Geometry check sheet. Reference: drawing and pictorial views, mm from the part's lowest x, y, z. A direction names the side the tool comes from. Coordinates: 2 decimals unless noted, no trailing zeros. Loops run counter-clockwise (first coordinate to the right, second up) from the corner with the lowest first, then second, coordinate; pieces in that order, holes last. Notation, with made-up numbers: (-11.5, -3.75) -> (46.5, -3.75) arc R25 cw to (46.5, 18.25) -> close; hole circle Ø9 at (64, 37.5). An arc over 180 degrees is marked (long way). Answer as a JSON object with one key per item and string values. Group by question number.
Q1. Cross-section at B-B on z = 5.5. Record the boundary of the cut face in (x, y).
Q2. Set-up check for the marked faces 1, 2, 3, 4 and 5: record each of +Z, -Z, +X, -X, +Y, -Y from which the full face is reachable in a straight line by a thin tool's end or side.
Q3. Cross-section at C-C on x = 25. Record the boundary of the cut face in (y, z).
Q4. Cross-section at A-A on y = 30.5. Record the boundary of the cut face in (x, z).
Q5. Scan lines: L1, parallel to X at y = 37, z = 5.5; L2, parallel to Y at x = 45, z = 5.6; L3, parallel to X at y = 38, z = 0.85. Record each from-to range of solid material in increasing order.
Q6. Gauge pin test, flat ends, axial feed: pin 1 Ø5 at (x, y) = (25, 15.5) entering from -Z; pin 2 Ø2 at (x, y) = (11, 33) entering from +Z; pin 3 Ø22.5 at (x, y) = (36, 30) entering from +Z. Record the tip position at first contact, or that the pin passes through.
Q7. Cross-section at D-D on y = 6. Record the boundary of the cut face in (x, z), and give its area (3 significant figures).
Q8. Release check for a two-part mould opening along Z. For the marked faces 6, 7 and 8 record: released by +Z, released by -Z, zero draft, split by the parting line, or undercut.
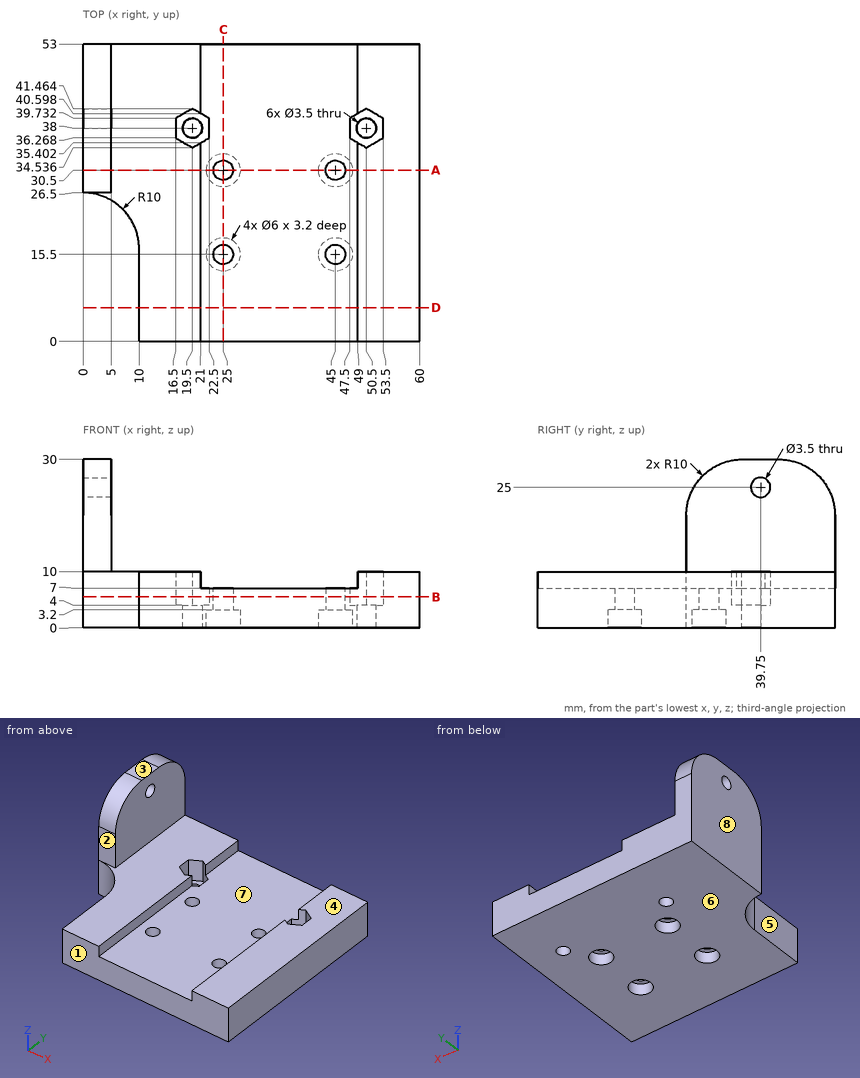
Computed values:
{
 "1": {"outline": "(0, 26.5) arc R10 cw to (10, 16.5) -> (10, 0) -> (60, 0) -> (60, 53) -> (0, 53) -> close; hole (16.5, 36.27) -> (19.5, 34.54) -> (22.5, 36.27) -> (22.5, 39.73) -> (19.5, 41.46) -> (16.5, 39.73) -> close; hole circle Ø3.5 at (25, 15.5); hole circle Ø3.5 at (25, 30.5); hole circle Ø3.5 at (45, 15.5); hole circle Ø3.5 at (45, 30.5); hole (47.5, 36.27) -> (50.5, 34.54) -> (53.5, 36.27) -> (53.5, 39.73) -> (50.5, 41.46) -> (47.5, 39.73) -> close"},
 "2": {"face 1": "+Z, -Z, +X, -X, -Y", "face 2": "+Z, +X, -X, -Y", "face 3": "+Z, +X, -X, +Y, -Y", "face 4": "+Z, +X, +Y, -Y", "face 5": "+Z, -Z, -X, -Y"},
 "3": {"outline": "(0, 0) -> (12.5, 0) -> (12.5, 3.2) -> (13.75, 3.2) -> (13.75, 7) -> (0, 7) -> close; (17.25, 3.2) -> (18.5, 3.2) -> (18.5, 0) -> (27.5, 0) -> (27.5, 3.2) -> (28.75, 3.2) -> (28.75, 7) -> (17.25, 7) -> close; (32.25, 3.2) -> (33.5, 3.2) -> (33.5, 0) -> (53, 0) -> (53, 7) -> (32.25, 7) -> close"},
 "4": {"outline": "(0, 0) -> (22, 0) -> (22, 3.2) -> (23.25, 3.2) -> (23.25, 7) -> (21, 7) -> (21, 10) -> (5, 10) -> (5, 28) -> (0, 28) -> close; (26.75, 3.2) -> (28, 3.2) -> (28, 0) -> (42, 0) -> (42, 3.2) -> (43.25, 3.2) -> (43.25, 7) -> (26.75, 7) -> close; (46.75, 3.2) -> (48, 3.2) -> (48, 0) -> (60, 0) -> (60, 10) -> (49, 10) -> (49, 7) -> (46.75, 7) -> close"},
 "5": {"L1": "x = 0 to 16.5, 22.5 to 47.5, 53.5 to 60", "L2": "y = 0 to 13.75, 17.25 to 28.75, 32.25 to 53", "L3": "x = 0 to 17.75, 21.25 to 48.75, 52.25 to 60"},
 "6": {"pin 1": "stops at z = 3.2", "pin 2": "stops at z = 10", "pin 3": "stops at z = 7"},
 "7": {"outline": "(10, 0) -> (60, 0) -> (60, 10) -> (49, 10) -> (49, 7) -> (21, 7) -> (21, 10) -> (10, 10) -> close", "area": "416 mm²"},
 "8": {"face 6": "released by -Z", "face 7": "released by +Z", "face 8": "zero draft"}
}
